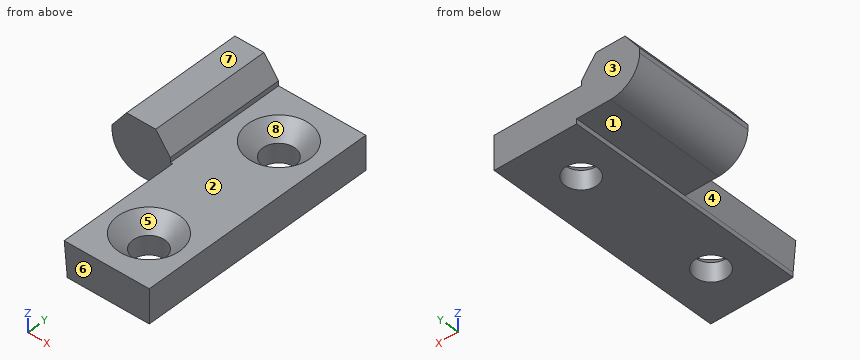
```python
from build123d import *

# Parameters (mm, degrees)
EXTRUDE_1_DEPTH           = 50
FILLET_1_R                = 6
HOLE_WIZARD_1_D           = 6.6
HOLE_WIZARD_1_CSINK_D     = 12.8
HOLE_WIZARD_1_CSINK_ANGLE = 90


with BuildPart() as part:
    # 草图1 → 凸台-拉伸1 (new body)
    with BuildSketch(Plane(origin=(0, 0, 0), x_dir=(1, 0, 0), z_dir=(0, 1, 0))):
        Polygon((0, 0), (-18, 0), (-18, -1), (-21, -5), (-27, -5), (-30, -1), (-30, 6), (-17, 6), (-17, 7), (0, 7), align=None)
    extrude(amount=EXTRUDE_1_DEPTH)

    # 圆角1
    fillet_1_edges = [part.edges().sort_by_distance(p)[0] for p in [
        (-30, 25, -6),
    ]]
    fillet(fillet_1_edges, radius=FILLET_1_R)

    # 打孔尺寸根据内六角花形半沉头螺钉的类型1 (through all)
    with Locations(Plane.XY):
        with Locations((-9, 40), (-9, 10)):
            CounterSinkHole(HOLE_WIZARD_1_D / 2, HOLE_WIZARD_1_CSINK_D / 2, counter_sink_angle=HOLE_WIZARD_1_CSINK_ANGLE)

    # 草图2 → 切除-放样1 section 0
    with BuildSketch(Plane.XY.offset(5)):
        with BuildLine():
            Line((-30, 0), (-18, 0))
            Line((-18, 0), (-18, 25))
            Line((-18, 25), (-30, 25))
            Line((-30, 25), (-30, 0))
        make_face()
    # 草图5 → 切除-放样1 section 1
    with BuildSketch(Plane(origin=(0, 0, -6), x_dir=(-1, 0, 0), z_dir=(0, 0, -1))):
        with BuildLine():
            Line((30, 25), (17, 25))
            Line((17, 25), (17, 0))
            Line((17, 0), (30, 0))
            Line((30, 0), (30, 25))
        make_face()
    loft(mode=Mode.SUBTRACT)


solid = part.part
```
Work out the finished part from the listing and answer in its coordinate system (mm). Face numbers are marked on the shaded views. A direction names the side the tool comes from. Give positions to 0.01 mm unless a question says otherwise; leave off trailing zeros. Loops run counter-clockwise (first coordinate to the right, second up) from the corner with the lowest first, then second, coordinate; pieces in that order, holes last. Notation, with made-up numbers: (-25, 8) - (14, 8) arc R23 cw to (14, 46) - close; hole circle Ø5 at (67.25, -2). An arc over 180 degrees is marked (long way). Use CSV: the item, a comma, the result in double quotes. Start each with the question number.
(1) Find section C-C, the plane y = 31.5. Determine the outline of the cut face in (x, z), plus the area to 3 significant figures.
(2) Determine the mould class of the marked faces 5, 6, 7 and 8 for opening direction Y: released by +Y, released by -Y, zero draft, split by the parting line, or undercut.
(3) Find section B-B, the plane x = -9. Determine the outline of the cut face in (y, z), plus the area to 3 significant figures.
(4) A tool of negligible diameter and unlimited length cuts with its end or side. For the marked faces 1, 2, 3 and 4, from which of +Z, -Z, +X, -X, +Y, -Y can it reach the whole face along a straight path? Write none if from no direction.
(5) Find section D-D, the plane y = 40. Determine the outline of the cut face in (x, z).
(6) Each of these flat-tipped pins is pushed along its axis until it touches: pin 1 (7.5 mm diameter, centred on x = -9, y = 40, fed in from +Z); pin 2 (1.5 mm diameter, centred on x = -6, z = 2.5, fed in from +Y); pin 3 (3 mm diameter, centred on x = -22, z = -5.5, fed in from -Y); pin 4 (0.8 mm diameter, centred on y = 36.5, z = 0.5, fed in from +X). Where does it stop, or does it pass through?
(7) Find the intervals of material crossed by L1, parallel to Y at x = -9, z = -5.85; L2, parallel to X at y = 40, z = -6.25; L3, parallel to Z at x = -21.5, y = 45, in increasing order.
(8) Find section A-A, the plane y = 10. Determine the outline of the cut face in (x, z), plus the area to 3 significant figures.
Results found:
1,outline,"(-30, 0) arc R6 ccw to (-24, -6) - (-17, -6) - (-17, -7) - (0, -7) - (0, 0) - (-18, 0) - (-18, 1) - (-21, 5) - (-27, 5) - (-30, 1) - close"
1,area,"237 mm^2"
2,face 5,"undercut"
2,face 6,"released by -Y"
2,face 7,"zero draft"
2,face 8,"undercut"
3,outline,"(0, -7) - (6.7, -7) - (6.7, -3.1) - (3.6, 0) - (0, 0) - close; (13.3, -7) - (36.7, -7) - (36.7, -3.1) - (33.6, 0) - (16.4, 0) - (13.3, -3.1) - close; (43.3, -7) - (50, -7) - (50, 0) - (46.4, 0) - (43.3, -3.1) - close"
3,area,"238 mm^2"
4,face 1,"-Z, -X, +Y, -Y"
4,face 2,"+Z, +X, +Y, -Y"
4,face 3,"+Z, -Z, +X, -X, +Y"
4,face 4,"-Z, -X, -Y"
5,outline,"(-30, 0) arc R6 ccw to (-24, -6) - (-17, -6) - (-17, -7) - (-12.3, -7) - (-12.3, -3.1) - (-15.4, 0) - (-18, 0) - (-18, 1) - (-21, 5) - (-27, 5) - (-30, 1) - close; (-5.7, -7) - (0, -7) - (0, 0) - (-2.6, 0) - (-5.7, -3.1) - close"
6,pin 1,"z = -2.65"
6,pin 2,"through"
6,pin 3,"y = 25"
6,pin 4,"x = -18"
7,L1,"0 to 6.7, 13.3 to 36.7, 43.3 to 50"
7,L2,"-17 to -12.3, -5.7 to 0"
7,L3,"-6 to 5"
8,outline,"(-17.55, 0) - (-17, -6) - (-17, -7) - (-12.3, -7) - (-12.3, -3.1) - (-15.4, 0) - close; (-5.7, -7) - (0, -7) - (0, 0) - (-2.6, 0) - (-5.7, -3.1) - close"
8,area,"64.8 mm^2"
